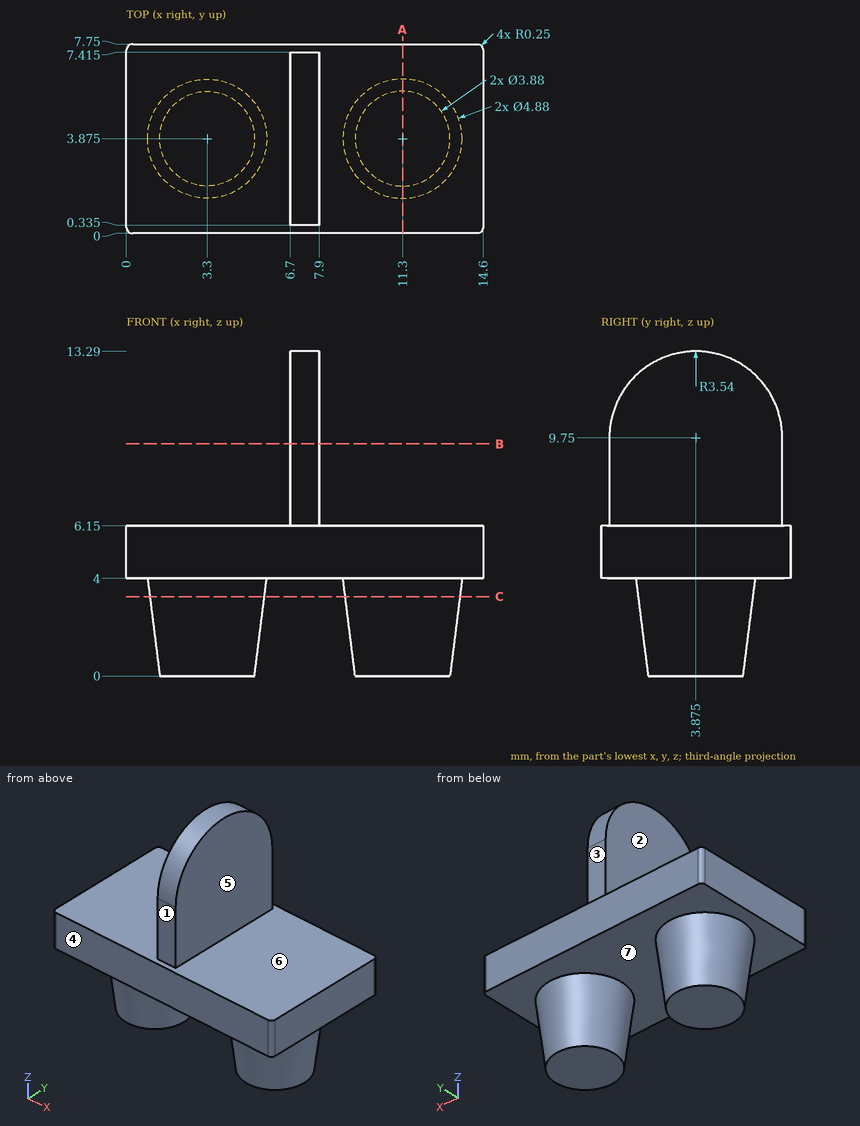
Here's the drawing with two shaded views (mm, measured from the low corner). I have some questions. A direction names the side the tool comes from. Coordinates: 2 decimals unless noted, no trailing zeros. Write each loop counter-clockwise with the first axis right and the second up, starting at its lowest first coordinate (ties: lowest second). Pieces come first, ordered by that corner, then holes.
Item 1: I want a section at C-C on z = 3.25. Write out the boundary of the cut face in (x, y) (1 decimal), and give its area (3 significant figures).
Item 2: I want a section at B-B on z = 9.5. Write out the boundary of the cut face in (x, y) (3 decimals).
Item 3: On a 3-axis mill with a long thin cutter (end or side, diameter ignored), from which of +Z, -Z, +X, -X, +Y, -Y can I reach the whole of each face in a straight line? I mean the marked faces 1, 2, 3 and 4. Say none if no direction works.
Item 4: I want a section at A-A on x = 11.3. Write out the boundary of the cut face in (y, z) (3 decimals).
Item 5: Will these pins go through, and if not, where does the flat tip stop? pin 1 (1.3 mm diameter, centred on x = 7, z = 8, fed in from +Y) (3 decimals); pin 2 (1.5 mm diameter, centred on y = 6.5, z = 10, fed in from +X); pin 3 (4 mm diameter, centred on y = 1.5, z = 10.5, fed in from -X).
Item 6: If I drill on line 1 (X direction, y = 4.5, z = 6.25); line 2 (Z direction, x = 2.75, y = 5); line 3 (Z direction, x = 13.5, y = 7.25), over which ranges is the centre line in solid material (lowest first)?
Item 7: If we mould it in two halves opening along X, with no side actions, what happens to the marked faces 5, 6 and 7? For each: +X half, -X half, draft (parallel to the pull), parting line (faces both ways), or undercut.
Findings below:
1. outline: circle Ø4.7 at (3.3, 3.9); circle Ø4.7 at (11.3, 3.9)
1. area: 34.6 mm2
2. outline: (6.7, 0.335) - (7.9, 0.335) - (7.9, 7.415) - (6.7, 7.415) - close
3. face 1: +Z, +X, -X, -Y
3. face 2: +Z, -X, +Y, -Y
3. face 3: +Z, +X, -X, +Y
3. face 4: +Z, -Z, +X, -X, -Y
4. outline: (0, 4) - (1.435, 4) - (1.935, 0) - (5.815, 0) - (6.315, 4) - (7.75, 4) - (7.75, 6.15) - (0, 6.15) - close
5. pin 1: stops at y = 7.415
5. pin 2: stops at x = 7.9
5. pin 3: stops at x = 6.7
6. line 1: x = 6.7 to 7.9
6. line 2: z = 0 to 6.15
6. line 3: z = 4 to 6.15
7. face 5: +X half
7. face 6: draft
7. face 7: undercut
